For this review, take the finished solid that the model builds, in its own axes (mm). A direction names the side the tool comes from. Give positions to 0.01 mm unless a question says otherwise; leave off trailing zeros. Order: outer loops, then holes, each group sorted by start corner. A loop starts at its lowest first (then second) coordinate and runs counter-clockwise, first axis right, second up.
from build123d import *

# Parameters (mm, degrees)
SKETCH_1_W          = 42
SKETCH_1_H          = 42
SKETCH_1_R          = 1.65
SKETCH_1_R_2        = 12.75
EXTRUDE_1_DEPTH     = 5
SKETCH_2_R          = 14.5
CUT_EXTRUDE_1_DEPTH = 2.5
CHAMFER_1_SIZE      = 4.2
SKETCH_3_R          = 1.95
CUT_EXTRUDE_2_DEPTH = 3.2
CHAMFER_2_SIZE      = 0.5
SKETCH_4_R          = 3
CUT_EXTRUDE_3_DEPTH = 3.3


with BuildPart() as part:
    # 草图1 → 凸台-拉伸1 (new body)
    with BuildSketch(Plane(origin=(0, 0, 0), x_dir=(1, 0, 0), z_dir=(0, 1, 0))):
        with Locations((21, 21)):
            Rectangle(SKETCH_1_W, SKETCH_1_H)
        with Locations((5.5, 5.5)):
            Circle(SKETCH_1_R, mode=Mode.SUBTRACT)
        with Locations((36.5, 5.5)):
            Circle(SKETCH_1_R, mode=Mode.SUBTRACT)
        with Locations((36.5, 36.5)):
            Circle(SKETCH_1_R, mode=Mode.SUBTRACT)
        with Locations((5.5, 36.5)):
            Circle(SKETCH_1_R, mode=Mode.SUBTRACT)
        with Locations((21, 21)):
            Circle(SKETCH_1_R_2, mode=Mode.SUBTRACT)
    extrude(amount=EXTRUDE_1_DEPTH)

    # 草图2 → 切除-拉伸1 (cut)
    with BuildSketch(Plane(origin=(0, 5, 0), x_dir=(1, 0, 0), z_dir=(0, 1, 0))):
        with Locations((21, 21)):
            Circle(SKETCH_2_R)
    extrude(amount=-CUT_EXTRUDE_1_DEPTH, mode=Mode.SUBTRACT)

    # 倒角1
    chamfer_1_edges = [part.edges().sort_by_distance(p)[0] for p in [
        (0, 2.5, -42),
        (42, 2.5, -42),
        (42, 2.5, 0),
        (0, 2.5, 0),
    ]]
    chamfer(chamfer_1_edges, length=CHAMFER_1_SIZE)

    # 草图3 → 切除-拉伸2 (cut)
    with BuildSketch(Plane.XZ):
        with Locations((38, -21)):
            Circle(SKETCH_3_R)
        with Locations((21, -38)):
            Circle(SKETCH_3_R)
        with Locations((4, -21)):
            Circle(SKETCH_3_R)
        with Locations((21, -4)):
            Circle(SKETCH_3_R)
    extrude(amount=-CUT_EXTRUDE_2_DEPTH, mode=Mode.SUBTRACT)

    # 倒角2
    chamfer_2_edges = [part.edges().sort_by_distance(p)[0] for p in [
        (36.05, 0, -21),
        (19.05, 0, -38),
        (2.05, 0, -21),
        (19.05, 0, -4),
    ]]
    chamfer(chamfer_2_edges, length=CHAMFER_2_SIZE)

    # 草图4 → 切除-拉伸3 (cut)
    with BuildSketch(Plane.XZ):
        with Locations((5.5, -5.5)):
            Circle(SKETCH_4_R)
        with Locations((36.5, -5.5)):
            Circle(SKETCH_4_R)
        with Locations((36.5, -36.5)):
            Circle(SKETCH_4_R)
        with Locations((5.5, -36.5)):
            Circle(SKETCH_4_R)
    extrude(amount=-CUT_EXTRUDE_3_DEPTH, mode=Mode.SUBTRACT)


solid = part.part
1) We need section A-A on x = 21. Give the boundary of the cut face in (y, z), then the cut area to 3 significant figures.
Answer sheet:
outline: (0, -42) - (5, -42) - (5, -35.5) - (2.5, -35.5) - (2.5, -33.75) - (0, -33.75) - (0, -35.55) - (0.5, -36.05) - (3.2, -36.05) - (3.2, -39.95) - (0.5, -39.95) - (0, -40.45) - close; (0, -8.25) - (2.5, -8.25) - (2.5, -6.5) - (5, -6.5) - (5, 0) - (0, 0) - (0, -1.55) - (0.5, -2.05) - (3.2, -2.05) - (3.2, -5.95) - (0.5, -5.95) - (0, -6.45) - close
area: 48.3 mm2
2) We need section B-B on z = -21. Give the boundary of the cut face in (x, y).
Answer sheet:
outline: (0, 0) - (1.55, 0) - (2.05, 0.5) - (2.05, 3.2) - (5.95, 3.2) - (5.95, 0.5) - (6.45, 0) - (8.25, 0) - (8.25, 2.5) - (6.5, 2.5) - (6.5, 5) - (0, 5) - close; (33.75, 0) - (35.55, 0) - (36.05, 0.5) - (36.05, 3.2) - (39.95, 3.2) - (39.95, 0.5) - (40.45, 0) - (42, 0) - (42, 5) - (35.5, 5) - (35.5, 2.5) - (33.75, 2.5) - close
3) Clearance check with a flat-ended pin moving along its axis: pin 1 (5 mm diameter, centred on x = 36.5, z = -36.5, fed in from -Y). State where the tip first meets the part, or that it passes through.
Answer sheet:
pin 1: stops at y = 3.3
4) Draft analysis for pull direction Z (two halves, no side actions). For faces 4 (the face through (0, 2, -21)), 5 (the face through (5.109, 1.627, -2.526)), 6 (the face through (2.1, 2.5, -39.9)), state which applies: +Z half, -Z half, draft (parallel to the pull), parting line (faces both ways), or undercut.
Answer sheet:
face 4: draft
face 5: undercut
face 6: -Z half
5) We need section C-C on y = 4.1. Give the boundary of the cut face in (x, z), then the cut area to 3 significant figures.
Answer sheet:
outline: (0, -37.8) - (4.2, -42) - (37.8, -42) - (42, -37.8) - (42, -4.2) - (37.8, 0) - (4.2, 0) - (0, -4.2) - close; hole circle Ø3.3 at (5.5, -36.5); hole circle Ø3.3 at (5.5, -5.5); hole circle Ø29 at (21, -21); hole circle Ø3.3 at (36.5, -36.5); hole circle Ø3.3 at (36.5, -5.5)
area: 1,030 mm2
6) To check wall thickness, follow line 1 (Z direction, x = 5.5, y = 3.8); line 2 (Z direction, x = 21, y = 1.9); line 3 (X direction, y = 4.4, z = -5.5). State the ranges of each line that lie inside material, in increasing order.
Answer sheet:
line 1: z = -42 to -38.15, -34.85 to -7.15, -3.85 to 0
line 2: z = -42 to -39.95, -36.05 to -33.75, -8.25 to -5.95, -2.05 to 0
line 3: x = 0 to 3.85, 7.15 to 34.85, 38.15 to 42
7) We need section D-D on x = 28. Give the boundary of the cut face in (y, z).
Answer sheet:
outline: (0, -42) - (5, -42) - (5, -33.7) - (2.5, -33.7) - (2.5, -31.66) - (0, -31.66) - close; (0, -10.34) - (2.5, -10.34) - (2.5, -8.3) - (5, -8.3) - (5, 0) - (0, 0) - close
8) Tool access review of faces 1 (the face through (33.5, 1.6, -36.4)), 2 (the face through (21, 2.5, -8)), 3 (the face through (34.85, 4.14, -5.57)): name each direction out of +Z, -Z, +X, -X, +Y, -Y from which nothing blocks a thin tool from reaching the whole face with its end or side.
Answer sheet:
face 1: -Y
face 2: +Y
face 3: +Y, -Y
